```python
from build123d import *

# Parameters (mm, degrees)
BOSS_EXTRUDE1_DEPTH = 3
BOSS_EXTRUDE2_DEPTH = 3
SKETCH3_R           = 2.25
BOSS_EXTRUDE3_DEPTH = 6.5
FILLET1_R           = 0.1
SKETCH6_R           = 1.5
CUT_EXTRUDE3_DEPTH  = 30.962406787
SKETCH7_R           = 2.25
CUT_EXTRUDE4_DEPTH  = 0.6
SKETCH8_R           = 0.75
CUT_EXTRUDE5_DEPTH  = 7


# Read off the part's stored shape, not the designer's step: Boss-Extrude2
with BuildPart() as part:
    # Sketch1 → Boss-Extrude1 (new body)
    with BuildSketch(Plane(origin=(0, 0, 0), x_dir=(1, 0, 0), z_dir=(0, 1, 0))):
        with BuildLine():
            Line((-23, 3), (-10.062305899, 3))
            ThreePointArc((-10.062305899, 3), (10.5, 0), (-10.062305899, -3))
            Line((-10.062305899, -3), (-23, -3))
            ThreePointArc((-23, -3), (-26, 0), (-23, 3))
        make_face()
    extrude(amount=BOSS_EXTRUDE1_DEPTH)

    # Boss-Extrude2 outline → Boss-Extrude2 (add)
    with BuildSketch(Plane(origin=(0, 0, 0), x_dir=(1, 0, 0), z_dir=(0, 1, 0))):
        with BuildLine():
            ThreePointArc((-5.522818211, -9.478178454), (-5.113524662, -9.318232563), (-4.681499231, -9.398593775))
            ThreePointArc((-4.681499231, -9.398593775), (-6.330495099, -8.377041948), (-7.763435591, -7.069587529))
            ThreePointArc((-7.763435591, -7.069587529), (-7.568178787, -7.463260843), (-7.61030601, -7.900672771))
            Line((-7.61030601, -7.900672771), (-8.279523298, -9.604618361))
            ThreePointArc((-8.279523298, -9.604618361), (-8.203196552, -10.651208986), (-7.156206429, -10.721844617))
            Line((-7.156206429, -10.721844617), (-5.522818211, -9.478178454))
        make_face()
        with BuildLine():
            ThreePointArc((-1.721512659, -10.833918126), (-1.397763446, -10.536788435), (-0.965920838, -10.455476887))
            ThreePointArc((-0.965920838, -10.455476887), (-2.872731946, -10.099376771), (-4.681499231, -9.398593775))
            ThreePointArc((-4.681499231, -9.398593775), (-4.357094721, -9.695015118), (-4.238192033, -10.118058909))
            Line((-4.238192033, -10.118058909), (-4.245930648, -11.948693352))
            ThreePointArc((-4.245930648, -11.948693352), (-3.796296521, -12.896853076), (-2.79461913, -12.584091002))
            Line((-2.79461913, -12.584091002), (-1.721512659, -10.833918126))
        make_face()
        with BuildLine():
            ThreePointArc((2.312803759, -10.723261005), (2.507193937, -10.329163724), (2.880407716, -10.097190272))
            ThreePointArc((2.880407716, -10.097190272), (0.973862068, -10.454740201), (-0.965920838, -10.455476887))
            ThreePointArc((-0.965920838, -10.455476887), (-0.556271486, -10.614522786), (-0.292428604, -10.965941515))
            Line((-0.292428604, -10.965941515), (0.362358895, -12.675484051))
            ThreePointArc((0.362358895, -12.675484051), (1.124441346, -13.396877181), (1.945226568, -12.7430505))
            Line((1.945226568, -12.7430505), (2.312803759, -10.723261005))
        make_face()
        with BuildLine():
            ThreePointArc((6.034076643, -9.161184796), (6.072796451, -8.723461012), (6.336866889, -8.372223004))
            ThreePointArc((6.336866889, -8.372223004), (4.688647545, -9.39502976), (2.880407716, -10.097190272))
            ThreePointArc((2.880407716, -10.097190272), (3.319847778, -10.097333864), (3.692915739, -10.329557645))
            Line((3.692915739, -10.329557645), (4.921602293, -11.686617593))
            ThreePointArc((4.921602293, -11.686617593), (5.892983381, -12.083601839), (6.421781187, -11.177207559))
            Line((6.421781187, -11.177207559), (6.034076643, -9.161184796))
        make_face()
        with BuildLine():
            ThreePointArc((8.938622786, -6.359120261), (8.816430498, -5.937014916), (8.935616531, -5.514050889))
            ThreePointArc((8.935616531, -5.514050889), (7.768814222, -7.063676492), (6.336866889, -8.372223004))
            ThreePointArc((6.336866889, -8.372223004), (6.746618445, -8.213446044), (7.178415082, -8.295043382))
            Line((7.178415082, -8.295043382), (8.814695021, -9.115939424))
            ThreePointArc((8.814695021, -9.115939424), (9.863895986, -9.134782017), (10.029132325, -8.098502778))
            Line((10.029132325, -8.098502778), (8.938622786, -6.359120261))
        make_face()
        with BuildLine():
            ThreePointArc((10.633304904, -2.696333552), (10.366740607, -2.346987899), (10.324902114, -1.909553962))
            ThreePointArc((10.324902114, -1.909553962), (9.797448349, -3.776242293), (8.935616531, -5.514050889))
            ThreePointArc((8.935616531, -5.514050889), (9.260219543, -5.217846902), (9.692298733, -5.13777511))
            Line((9.692298733, -5.13777511), (11.514697643, -5.311396998))
            ThreePointArc((11.514697643, -5.311396998), (12.499706621, -4.949547548), (12.279016357, -3.923646229))
            Line((12.279016357, -3.923646229), (10.633304904, -2.696333552))
        make_face()
        with BuildLine():
            Line((12.95822192, 0.637416485), (10.427354789, 1.23299315))
            ThreePointArc((10.427354789, 1.23299315), (10.49442434, -0.342137064), (10.324902114, -1.909553962))
            ThreePointArc((10.324902114, -1.909553962), (10.520420766, -1.516004291), (10.894306512, -1.285096658))
            Line((10.894306512, -1.285096658), (12.870116963, -0.727570251))
            ThreePointArc((12.870116963, -0.727570251), (13.298325237, -0.06987275), (12.95822192, 0.637416485))
        make_face()
    extrude(amount=BOSS_EXTRUDE2_DEPTH)

    # Sketch5 → Revolve1 (revolve)
    with BuildSketch(Plane.XY, mode=Mode.PRIVATE) as revolve1_sk:
        Polygon((-3.7, 8), (-6.789097331, 8), (-9.5, 3), (-1.5, 3), (-1.5, 6), (-3.7, 6), align=None)
    revolve(revolve1_sk.sketch.rotate(Axis((0, 0, 0), (0, 1, 0)), 270), axis=Axis((0, 0, 0), (0, 1, 0)))

    # Sketch3 → Boss-Extrude3 (add)
    with BuildSketch(Plane(origin=(0, 3, 0), x_dir=(1, 0, 0), z_dir=(0, 1, 0))):
        with Locations(Location((-23, 0, 0), (0, 0, 90))):
            Circle(SKETCH3_R)
    extrude(amount=BOSS_EXTRUDE3_DEPTH)

    # Fillet1
    fillet1_edges = [part.edges().sort_by_distance(p)[0] for p in [
        (-23, 9.5, 2.25),
    ]]
    fillet(fillet1_edges, radius=FILLET1_R)

    # Sketch6 → Cut-Extrude3 (cut, through all)
    with BuildSketch(Plane(origin=(0, 3, 0), x_dir=(1, 0, 0), z_dir=(0, 1, 0))):
        with Locations(Location((0, 0, 0), (0, 0, 90))):
            Circle(SKETCH6_R)
    extrude(amount=-CUT_EXTRUDE3_DEPTH, mode=Mode.SUBTRACT)

    # Sketch7 → Cut-Extrude4 (cut)
    with BuildSketch(Plane(origin=(0, 0, 0), x_dir=(1, 0, 0), z_dir=(0, 1, 0))):
        with Locations(Location((-23, 0, 0), (0, 0, 90))):
            Circle(SKETCH7_R)
    extrude(amount=CUT_EXTRUDE4_DEPTH, mode=Mode.SUBTRACT)

    # Sketch8 → Cut-Extrude5 (cut)
    with BuildSketch(Plane.XZ.offset(-0.6)):
        with Locations(Location((-23, 0, 0), (0, 0, 270))):
            Circle(SKETCH8_R)
    extrude(amount=-CUT_EXTRUDE5_DEPTH, mode=Mode.SUBTRACT)


solid = part.part
```
The model under review builds one solid part; all positions refer to its coordinate system, in mm. A direction names the side the tool comes from. Give positions to 0.01 mm unless a question says otherwise; leave off trailing zeros. Write each loop counter-clockwise with the first axis right and the second up, starting at its lowest first coordinate (ties: lowest second). Pieces come first, ordered by that corner, then holes. Notation, with made-up numbers: (56, 33) -> (103, 33) arc R17 cw to (103, 51) -> close; hole circle Ø8 at (1.5, 57.5). An arc over 180 degrees is marked (long way). Put each result on its own line as item: value.
(1) Tool access review of faces 1 (the cylindrical face through (-9.126, 1.479, 5.193)), 2 (the flat face through (10.591, 1.479, 5.223)), 3 (the flat face through (2.126, 1.479, 11.747)), 4 (the flat face through (-16, 1, 3)), 5 (the flat face through (-24, 0.6, 1)): name each direction out of +Z, -Z, +X, -X, +Y, -Y from which nothing blocks a thin tool from reaching the whole face with its end or side.
Results are:
face 1: -X, +Y, -Y
face 2: +Y, -Y
face 3: +Z, +Y, -Y
face 4: +Z, -X, +Y, -Y
face 5: -Y
(2) We need section B-B, the plane y = 9. Give the boundary of the cut face in (x, z), and give its area (3 significant figures).
Results are:
outline: circle Ø4.5 at (-23, 0)
area: 15.9 mm²
(3) We need section C-C, the plane y = 4. Give the boundary of the cut face in (x, z), and give its area (3 significant figures).
Results are:
outline: circle Ø4.5 at (-23, 0); circle Ø17.92 at (0, 0); hole circle Ø1.5 at (-23, 0); hole circle Ø3 at (0, 0)
area: 259 mm²
(4) For pin 1 Ø4 at (y, z) = (7.5, -2.5) entering from +X; pin 2 Ø4 at (x, z) = (0, 0) entering from +Y; pin 3 Ø3.5 at (x, y) = (-16, 1) entering from -Z, all flat-tipped, find the tip position at first contact; note any pin that passes through.
Results are:
pin 1: x = 7.87
pin 2: y = 6
pin 3: z = -3
(5) The part is to be moulded in two halves that separate along Z. For faces 6 (the cylindrical face through (-26, 1, 0)), 7 (the flat face through (6.23, 1.48, 10.18)), 8 (the flat face through (0.03, 1.48, 11.81)), say which applies: pulls with the +Z half, pulls with the -Z half, needs draft (parallel to the pull), parting line crosses it, or undercut.
Results are:
face 6: parting line crosses it
face 7: undercut
face 8: pulls with the +Z half
(6) We need section D-D, the plane y = 7. Give the boundary of the cut face in (x, z).
Results are:
outline: circle Ø4.5 at (-23, 0); circle Ø14.66 at (0, 0); hole circle Ø1.5 at (-23, 0); hole circle Ø7.4 at (0, 0)
(7) To check wall thickness, follow probe 1 along X at (y, z) = (0.25, 0); probe 2 along X at (y, z) = (4.25, 0); probe 3 along Z at (x, y) = (-23, 0.3). State the ranges of each line that lie inside material, in increasing order. Write a range as from..to.
Results are:
probe 1: -26..-25.25, -20.75..-1.5, 1.5..13.3
probe 2: -25.25..-23.75, -22.25..-20.75, -8.82..-1.5, 1.5..8.82
probe 3: -3..-2.25, 2.25..3
